```python
from build123d import *

# Parameters (mm, degrees)
SKETCH1_W      = 780
SKETCH1_H      = 560
EXTRUDE1_DEPTH = 440
EXTRUDE1_TAPER = 2
SHELL1_T       = -5


with BuildPart() as part:
    # Sketch1 → Extrude1 (new body)
    with BuildSketch(Plane(origin=(0, 0, 0), x_dir=(1, 0, 0), z_dir=(0, 1, 0))):
        Rectangle(SKETCH1_W, SKETCH1_H)
    extrude(amount=-EXTRUDE1_DEPTH, taper=EXTRUDE1_TAPER)

    # Shell1
    shell1_openings = [part.faces().sort_by_distance(p)[0] for p in [
        (0, 0, 0),
    ]]
    offset(amount=SHELL1_T, openings=shell1_openings, kind=Kind.INTERSECTION)


solid = part.part
```
The listing builds one solid part. Answer for the finished solid, in the listing's coordinates (mm). Coordinates: 2 decimals unless noted, no trailing zeros. Return JSON: item names as keys, results as strings. Group by question number.
1. Given pin 1 (4 mm diameter, centred on y = -328.5, z = 174.5, fed in from -X); pin 2 (10 mm diameter, centred on x = 106, y = -198, fed in from +Z); pin 3 (3 mm diameter, centred on x = -89.5, z = -215, fed in from +Y), each flat-ended and moving along its own axis, determine where each tip first touches the part or whether it passes through.
2. Determine the mould class of faces 1 (the flat face through (-9, -435, -1)), 2 (the flat face through (-9, -440, -1)) for opening direction Z: released by +Z, released by -Z, zero draft, split by the parting line, or undercut.
3. Straight lines are drawn through the part: L1, parallel to Y at x = -321, z = 57.5; L2, parallel to Z at x = 212, y = -350; L3, parallel to Z at x = -327, y = -289. For each, find the intervals that lie inside material, in ascending order.
Ans:
{
 "1": {"pin 1": "x = -378.6", "pin 2": "z = 273.26", "pin 3": "y = -435"},
 "2": {"face 1": "undercut", "face 2": "zero draft"},
 "3": {"L1": "-440 to -435", "L2": "-267.78 to -262.77, 262.77 to 267.78", "L3": "-269.91 to -264.9, 264.9 to 269.91"}
}
